Here's how the part is built. I have some questions about the finished solid (model axes, mm). A direction names the side the tool comes from. Coordinates: 2 decimals unless noted, no trailing zeros. Order: outer loops, then holes, each group sorted by start corner. A loop starts at its lowest first (then second) coordinate and runs counter-clockwise, first axis right, second up. Notation, with made-up numbers: (16, -2) - (64, -2) arc R25 cw to (64, 17) - close; hole circle Ø1 at (85.5, 58.25). An arc over 180 degrees is marked (long way). Answer as CSV lines item,"result". Start each with the question number.
Q1. Suppose I cut it at C-C (y = -3). Please give me the cut outline in (x, z), then the cut area to 3 significant figures.
Q2. Suppose I cut it at B-B (z = -11.75). Please give me the cut outline in (x, y), then the cut area to 3 significant figures.
Q3. Thinking about a two-plate mould opening in X: for faces 1 (the face through (32.766, -14.479, -12.358)), 2 (the face through (1.5, -15, 0)), 3 (the face through (-10, -14, 0)), 4 (the face through (75, -14, 16)), which applies, released by +X, released by -X, zero draft, split by the parting line, or undercut?
Q4. I need wall thicknesses on line 1 (Z direction, x = 31.3, y = -14.45); line 2 (Y direction, x = 119, z = -5); line 3 (X direction, y = -1.25, z = 2.5). Which ranges of each line are inside material? Lowest first, please.
Q5. For faces 5 (the face through (0, -6, -3)), 6 (the face through (102.766, -14.479, 11.142)), 7 (the face through (-1.5, -15, 0)), which set-ups out of +Z, -Z, +X, -X, +Y, -Y let a thin tool reach every point of the face, with its end or its side?
Q6. Suppose I cut it at A-A (z = 0). Please give me the cut outline in (x, y), then the cut area to 3 significant figures.
Q7. Suppose I cut it at D-D (x = 71.5). Please give me the cut outline in (y, z).
Q8. For pin 1 Ø5 at (x, z) = (66.3, 11.75) entering from +Y; pin 2 Ø8 at (y, z) = (-5.5, -8.5) entering from -X, each with a flat end and sliding along its axis, tell me the tip position at first contact or that it passes through.
from build123d import *

# Parameters (mm, degrees)
SKETCH1_R           = 6
SKETCH1_R_2         = 3
BOSS_EXTRUDE1_DEPTH = 13
SKETCH2_W           = 171.5
SKETCH2_H           = 32
SKETCH2_R           = 1.5875
BOSS_EXTRUDE2_DEPTH = 3
CUT_EXTRUDE1_DEPTH  = 1.5


with BuildPart() as part:
    # Sketch1 → Boss-Extrude1 (new body)
    with BuildSketch(Plane(origin=(0, 0, 0), x_dir=(1, 0, 0), z_dir=(0, 1, 0))):
        Circle(SKETCH1_R)
        Circle(SKETCH1_R_2, mode=Mode.SUBTRACT)
    extrude(amount=-BOSS_EXTRUDE1_DEPTH)


with BuildPart() as body_2:
    # Sketch2 → Boss-Extrude2 (new body)
    with BuildSketch(Plane.XZ.offset(13)):
        with Locations((75.75, 0)):
            Rectangle(SKETCH2_W, SKETCH2_H)
        with Locations((136.3, -11.75)):
            Circle(SKETCH2_R, mode=Mode.SUBTRACT)
        with Locations((136.3, 11.75)):
            Circle(SKETCH2_R, mode=Mode.SUBTRACT)
        with Locations((101.3, -11.75)):
            Circle(SKETCH2_R, mode=Mode.SUBTRACT)
        with Locations((66.3, -11.75)):
            Circle(SKETCH2_R, mode=Mode.SUBTRACT)
        with Locations((31.3, -11.75)):
            Circle(SKETCH2_R, mode=Mode.SUBTRACT)
        with Locations((101.3, 11.75)):
            Circle(SKETCH2_R, mode=Mode.SUBTRACT)
        with Locations((66.3, 11.75)):
            Circle(SKETCH2_R, mode=Mode.SUBTRACT)
        with Locations((31.3, 11.75)):
            Circle(SKETCH2_R, mode=Mode.SUBTRACT)
        with Locations((-6.7, 11.75)):
            Circle(SKETCH2_R, mode=Mode.SUBTRACT)
        with Locations((-6.7, -11.75)):
            Circle(SKETCH2_R, mode=Mode.SUBTRACT)
    extrude(amount=BOSS_EXTRUDE2_DEPTH)


with BuildPart() as cut_extrude1_tool:
    # Sketch7 → Cut-Extrude1 (new body, symmetric)
    with BuildSketch(Plane.ZY):
        with BuildLine():
            ThreePointArc((-3, -11.395656787), (-3.439916375, -12.647111574), (-4.566139084, -13.348030908))
            Line((-4.566139084, -13.348030908), (-5.933860916, -13.651969092))
            ThreePointArc((-5.933860916, -13.651969092), (-7.060083625, -14.352888426), (-7.5, -15.604343213))
            Line((-7.5, -15.604343213), (-7.5, -16))
            Line((-7.5, -16), (7.5, -16))
            Line((7.5, -16), (7.5, -15.604343213))
            ThreePointArc((7.5, -15.604343213), (7.060083625, -14.352888426), (5.933860916, -13.651969092))
            Line((5.933860916, -13.651969092), (4.566139084, -13.348030908))
            ThreePointArc((4.566139084, -13.348030908), (3.439916375, -12.647111574), (3, -11.395656787))
            Line((3, -11.395656787), (-3, -11.395656787))
        make_face()
    extrude(amount=CUT_EXTRUDE1_DEPTH, both=True)


with BuildPart() as part_1:
    add(part.part)

    # Cut-Extrude1: cut by cut_extrude1_tool
    add(cut_extrude1_tool.part, mode=Mode.SUBTRACT)



with BuildPart() as body_2_1:
    add(body_2.part)

    # Cut-Extrude1: cut by cut_extrude1_tool
    add(cut_extrude1_tool.part, mode=Mode.SUBTRACT)


with BuildPart() as part_2:
    add(part_1.part)

    add(body_2_1.part)  # Revolve1 merges body 2
    # Sketch8 → Revolve1 (revolve)
    with BuildSketch(Plane.ZY):
        with BuildLine():
            Line((-8, -13), (-6, -13))
            Line((-6, -13), (-6, -11))
            ThreePointArc((-6, -11), (-6.585786438, -12.414213562), (-8, -13))
        make_face()
    revolve(axis=Axis((0, 4.095579303, 0), (0, -1, 0)))


solid = part_2.part
Here are the results:
1,outline,"circle Ø12 at (0, 0); hole circle Ø6 at (0, 0)"
1,area,"84.8 mm²"
2,outline,"(-10, -16) - (-8.29, -16) - (-8.29, -13) - (-10, -13) - close; (-5.11, -16) - (29.71, -16) - (29.71, -13) - (-5.11, -13) - close; (32.89, -16) - (64.71, -16) - (64.71, -13) - (32.89, -13) - close; (67.89, -16) - (99.71, -16) - (99.71, -13) - (67.89, -13) - close; (102.89, -16) - (134.71, -16) - (134.71, -13) - (102.89, -13) - close; (137.89, -16) - (161.5, -16) - (161.5, -13) - (137.89, -13) - close"
2,area,"467 mm²"
3,face 1,"undercut"
3,face 2,"undercut"
3,face 3,"released by -X"
3,face 4,"zero draft"
4,line 1,"z = -16 to -13.34, -10.16 to 10.16, 13.34 to 16"
4,line 2,"y = -16 to -13"
4,line 3,"x = -5.45 to -1.66, 1.66 to 5.45"
5,face 5,"+Y"
5,face 6,"+Y, -Y"
5,face 7,"-Y"
6,outline,"(-10, -16) - (-1.5, -16) - (-1.5, -13) - (-3, -13) - (-3, 0) - (-6, 0) - (-6, -11) arc R2 cw to (-8, -13) - (-10, -13) - close; (1.5, -16) - (161.5, -16) - (161.5, -13) - (8, -13) arc R2 cw to (6, -11) - (6, 0) - (3, 0) - (3, -13) - (1.5, -13) - close"
6,area,"585 mm²"
7,outline,"(-16, -16) - (-13, -16) - (-13, 16) - (-16, 16) - close"
8,pin 1,"stops at y = -13"
8,pin 2,"stops at x = -3.97"
